For this review, take the finished solid that the model builds, in its own axes (mm). Give positions to 0.01 mm unless a question says otherwise; leave off trailing zeros. Write each loop counter-clockwise with the first axis right and the second up, starting at its lowest first coordinate (ties: lowest second). Pieces come first, ordered by that corner, then holes. Notation, with made-up numbers: (-8, -3.75) -> (46, -3.75) arc R28 cw to (46, 27.25) -> close; hole circle Ø10 at (2, 39). An arc over 180 degrees is marked (long way). Write item = value, one per line.
```python
from build123d import *

# Parameters (mm, degrees)
SKETCH1_R          = 76
CIRCLE_DEPTH       = 5
SKETCH2_W          = 100
SKETCH2_H          = 100
SQUARE_DEPTH       = 5
SKETCH3_R          = 2.5
HOLES_DEPTH        = 5
CUT_EXTRUDE3_DEPTH = 5


with BuildPart() as part:
    # Sketch1 → circle (new body)
    with BuildSketch(Plane.XY):
        Circle(SKETCH1_R)
    extrude(amount=CIRCLE_DEPTH)

    # Sketch2 → square (cut)
    with BuildSketch(Plane.XY.offset(5)):
        Rectangle(SKETCH2_W, SKETCH2_H)
    extrude(amount=-SQUARE_DEPTH, mode=Mode.SUBTRACT)

    # Sketch3 → holes (cut)
    with BuildSketch(Plane.XY.offset(5)):
        with Locations((0, 60)):
            Circle(SKETCH3_R)
        with Locations((0, -60)):
            Circle(SKETCH3_R)
    extrude(amount=-HOLES_DEPTH, mode=Mode.SUBTRACT)

    # Sketch4 → Cut-Extrude3 (cut)
    with BuildSketch(Plane.XY.offset(5)):
        Polygon((-50, 0), (-50, -8.3), (-57.55, -8.3), (-60.903744176, -10), (-67.80719259, -6.5), (-67.80719259, 6.5), (-60.903744176, 10), (-57.55, 8.3), (-50, 8.3), align=None)
        Polygon((57.55, 8.3), (50, 8.3), (50, 0), (50, -8.3), (57.55, -8.3), (60.903744176, -10), (67.80719259, -6.5), (67.80719259, 6.5), (60.903744176, 10), align=None)
    extrude(amount=-CUT_EXTRUDE3_DEPTH, mode=Mode.SUBTRACT)


solid = part.part
```
(1) For pin 1 (1 mm diameter, centred on x = -13.5, z = 1, fed in from -Y); pin 2 (2 mm diameter, centred on y = 30.5, z = 1, fed in from +X); pin 3 (3 mm diameter, centred on y = 54, z = 3.5, fed in from +X); pin 4 (4.5 mm diameter, centred on x = 0, y = 60, fed in from +Z), all flat-tipped, find the tip position at first contact; note any pin that passes through.
Answers below:
pin_1 = -74.88
pin_2 = 70.04
pin_3 = 54.95
pin_4 = through
(2) Take a section at D-D (z = 3.05). Write out the cut boundary in (x, y).
Answers below:
outline = circle Ø152 at (0, 0); hole (-67.81, -6.5) -> (-60.9, -10) -> (-57.55, -8.3) -> (-50, -8.3) -> (-50, -50) -> (50, -50) -> (50, -8.3) -> (57.55, -8.3) -> (60.9, -10) -> (67.81, -6.5) -> (67.81, 6.5) -> (60.9, 10) -> (57.55, 8.3) -> (50, 8.3) -> (50, 50) -> (-50, 50) -> (-50, 8.3) -> (-57.55, 8.3) -> (-60.9, 10) -> (-67.81, 6.5) -> close; hole circle Ø5 at (0, -60); hole circle Ø5 at (0, 60)
(3) Take a section at B-B (y = 0). Write out the cut boundary in (x, z).
Answers below:
outline = (-76, 0) -> (-67.81, 0) -> (-67.81, 5) -> (-76, 5) -> close; (67.81, 0) -> (76, 0) -> (76, 5) -> (67.81, 5) -> close
(4) To check wall thickness, follow probe 1 along Y at (x, z) = (0, 2); probe 2 along Y at (x, z) = (-2, 2.4); probe 3 along X at (y, z) = (-18, 4.5). State the ranges of each line that lie inside material, in increasing order.
Answers below:
probe_1 = -76 to -62.5, -57.5 to -50, 50 to 57.5, 62.5 to 76
probe_2 = -75.97 to -61.5, -58.5 to -50, 50 to 58.5, 61.5 to 75.97
probe_3 = -73.84 to -50, 50 to 73.84
(5) Take a section at A-A (x = 0). Write out the cut boundary in (y, z), plus the area to 3 significant figures.
Answers below:
outline = (-76, 0) -> (-62.5, 0) -> (-62.5, 5) -> (-76, 5) -> close; (-57.5, 0) -> (-50, 0) -> (-50, 5) -> (-57.5, 5) -> close; (50, 0) -> (57.5, 0) -> (57.5, 5) -> (50, 5) -> close; (62.5, 0) -> (76, 0) -> (76, 5) -> (62.5, 5) -> close
area = 210 mm^2
(6) The part is to be moulded in two halves that separate along Y. For faces 1 (the face through (35.069, -67.425, 2.465)), 2 (the face through (10.9, -50.3, 5)), 3 (the face through (-64.404, 8.226, 2.535)), say which applies: released by +Y, released by -Y, zero draft, split by the parting line, or undercut.
Answers below:
face_1 = split by the parting line
face_2 = zero draft
face_3 = undercut
(7) Take a section at C-C (x = -38). Write out the cut boundary in (y, z).
Answers below:
outline = (-65.82, 0) -> (-50, 0) -> (-50, 5) -> (-65.82, 5) -> close; (50, 0) -> (65.82, 0) -> (65.82, 5) -> (50, 5) -> close
